Source: CAD feature listing. Evaluate the final solid. Frame: model axes, mm. Give positions to 0.01 mm unless a question says otherwise; leave off trailing zeros. Loops run counter-clockwise (first coordinate to the right, second up) from the corner with the lowest first, then second, coordinate; pieces in that order, holes last. Notation, with made-up numbers: M 23,75 L 59,75 A35 cw 59,111 Z; hole C 76,-32.75 d11. An arc over 180 degrees is marked long. Write item = value, one per line.
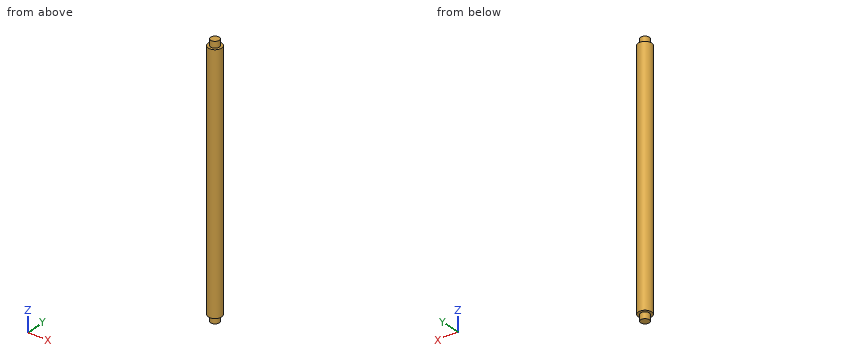
Autodesk Inventor part; units mm, degrees
ref_plane "YZ Plane" through (0, 0, 0) normal (1, 0, 0) x (0, 1, 0)
ref_plane "XZ Plane" through (0, 0, 0) normal (0, 1, 0) x (-1, 0, 0)
ref_plane "XY Plane" through (0, 0, 0) normal (0, 0, 1) x (1, 0, 0)
sketch "Sketch1" plane through (0, 0, 0) normal (0, 0, 1) x (1, 0, 0)
  circle A0 centre (0, 0) radius 9.5
  dimension "d0" = 19
extrude "Extrusion1" add sketch "Sketch1" along normal mid plane 350
sketch "Sketch2" plane through (0, 0, 175) normal (0, 0, 1) x (1, 0, 0)
  circle A0 centre (0, 0) radius 9.5
  circle A1 centre (0, 0) radius 6
  dimension "d3" = 12
extrude "Extrusion2" add sketch "Sketch2" along normal blind 9 contours A1
sketch "Sketch3" plane through (0, 0, -175) normal (0, 0, -1) x (-1, 0, 0)
  circle A0 centre (0, 0) radius 9.5
  circle A1 centre (0, 0) radius 6
  dimension "d6" = 12
extrude "Extrusion3" add sketch "Sketch3" along normal blind 9 contours A1
properties part number "ADSK-MH-10044" material "Steel, Mild"
1. Cut plane C-C, the plane z = -141.5. Return the cut outline in (x, y).
Derived:
outline = C 0,0 d19
2. Cut plane A-A, the plane x = 0. Return the cut outline in (y, z).
Derived:
outline = M -9.5,-175 L -6,-175 L -6,-184 L 6,-184 L 6,-175 L 9.5,-175 L 9.5,175 L 6,175 L 6,184 L -6,184 L -6,175 L -9.5,175 Z
3. First-contact query: pin 1 Ø5 at (y, z) = (6, 81) entering from +X; pin 2 Ø3 at (y, z) = (-2, 124.5) entering from +X. Flat tips, straight axial feed; report the tip coordinate or a pass-through.
Derived:
pin_1 = 8.83
pin_2 = 9.49
4. Material intervals for probe 1 along Z at (x, y) = (-6.5, 3); probe 2 along Y at (x, z) = (0.5, -112.5); probe 3 along X at (y, z) = (6.75, -37), sorted ascending. Write a range as from..to.
Derived:
probe_1 = -175..175
probe_2 = -9.49..9.49
probe_3 = -6.68..6.68
